Study the drawing (mm; zero at the part's minimum x, y, z) and answer. A direction names the side the tool comes from. Give positions to 0.01 mm unless a question says otherwise; leave off trailing zeros. Order: outer loops, then holes, each group sorted by start corner. A loop starts at its lowest first (then second) coordinate and runs counter-clockwise, first axis right, second up.
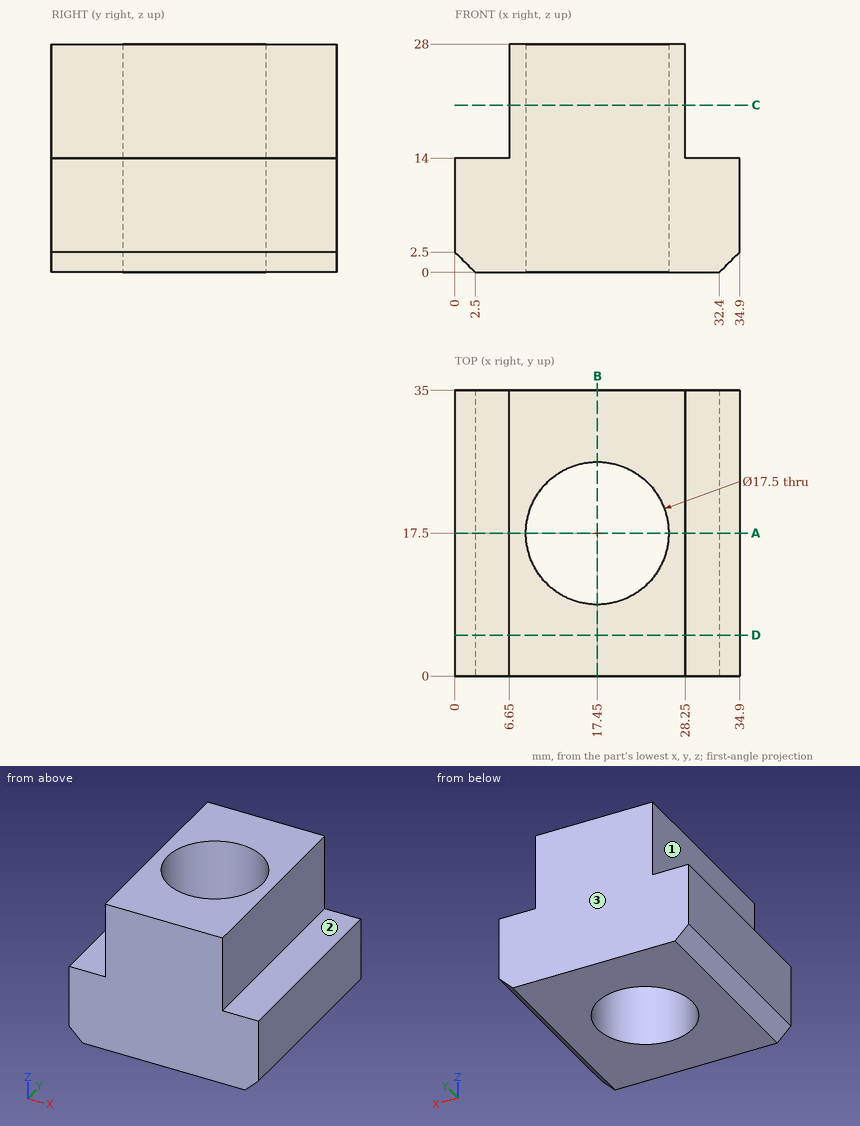
1) Find section D-D (y = 5). Write down the section's boundary in (x, z), then the cut area to 3 significant figures.
Geometry says:
outline: (0, 2.5) - (2.5, 0) - (32.4, 0) - (34.9, 2.5) - (34.9, 14) - (28.25, 14) - (28.25, 28) - (6.65, 28) - (6.65, 14) - (0, 14) - close
area: 785 mm2
2) A tool of negligible diameter and unlimited length cuts with its end or side. For the marked faces 1, 2 and 3, from which of +Z, -Z, +X, -X, +Y, -Y can it reach the whole face along a straight path? Write none if from no direction.
Geometry says:
face 1: +Z, -X, +Y, -Y
face 2: +Z, +X, +Y, -Y
face 3: +Z, -Z, +X, -X, +Y
3) Find section B-B (x = 17.45). Write down the section's boundary in (y, z).
Geometry says:
outline: (0, 0) - (8.75, 0) - (8.75, 28) - (0, 28) - close; (26.25, 0) - (35, 0) - (35, 28) - (26.25, 28) - close
4) Find section C-C (z = 20.5). Write down the section's boundary in (x, y), then the cut area to 3 significant figures.
Geometry says:
outline: (6.65, 0) - (28.25, 0) - (28.25, 35) - (6.65, 35) - close; hole circle Ø17.5 at (17.45, 17.5)
area: 515 mm2
5) Find section A-A (y = 17.5). Write down the section's boundary in (x, z), then the cut area to 3 significant figures.
Geometry says:
outline: (0, 2.5) - (2.5, 0) - (8.7, 0) - (8.7, 28) - (6.65, 28) - (6.65, 14) - (0, 14) - close; (26.2, 0) - (32.4, 0) - (34.9, 2.5) - (34.9, 14) - (28.25, 14) - (28.25, 28) - (26.2, 28) - close
area: 295 mm2
6) Straight lines are drawn through the part: probe 1 along Y at (x, z) = (17.45, 18.25); probe 2 along X at (y, z) = (31, 22.75); probe 3 along Y at (x, z) = (22, 18.5). For each, find the intervals that lie inside material, in ascending order.
Geometry says:
probe 1: y = 0 to 8.75, 26.25 to 35
probe 2: x = 6.65 to 28.25
probe 3: y = 0 to 10.03, 24.97 to 35
7) Given P1, Ø2, axis at x = 30, y = 17.5, coming from the +Z side; P2, Ø5, axis at y = 15.5, z = 19.5, coming from the -X side, each flat-ended and moving along its own axis, determine where each tip first touches the part or whether it passes through.
Geometry says:
P1: stops at z = 14
P2: stops at x = 6.65
